```python
from build123d import *

# Parameters (mm, degrees)
BOSS_EXTRUDE1_DEPTH      = 6.35
FILLET1_R                = 12.7
CUT_EXTRUDE2_DEPTH       = 3.175
BOSS_EXTRUDE2_DEPTH      = 3.175
BOSS_EXTRUDE2_DEPTH_BACK = 36.135303
SKETCH4_R                = 9.525
SKETCH4_R_2              = 6.35
SKETCH5_R                = 9.525
SKETCH5_R_2              = 6.35
BOSS_EXTRUDE3_DEPTH      = 25.4
CHAMFER2_SIZE            = 1
CHAMFER4_SIZE            = 1


with BuildPart() as part:
    # Sketch1 → Boss-Extrude1 (new, symmetric)
    with BuildSketch(Plane.YZ):
        Polygon((-25.4, 10.735303163), (0, 25.4), (25.4, 25.4), (25.4, -25.4), (-25.4, -25.4), align=None)
    extrude(amount=BOSS_EXTRUDE1_DEPTH, both=True)

    # Fillet1
    fillet1_edges = [part.edges().sort_by_distance(p)[0] for p in [
        (0, 25.4, -25.4),
    ]]
    fillet(fillet1_edges, radius=FILLET1_R)

    # Sketch3 → Cut-Extrude2 (cut)
    with BuildSketch(Plane.YZ.offset(6.35)):
        with BuildLine():
            Line((-22.225, -22.225), (12.7, -22.225))
            ThreePointArc((12.7, -22.225), (19.435192091, -19.435192091), (22.225, -12.7))
            Line((22.225, -12.7), (22.225, 22.225))
            Line((22.225, 22.225), (0.850738686, 22.225))
            Line((0.850738686, 22.225), (-22.225, 8.902216058))
            Line((-22.225, 8.902216058), (-22.225, -22.225))
        make_face()
    cut_extrude2 = extrude(amount=-CUT_EXTRUDE2_DEPTH, mode=Mode.SUBTRACT)

    # Mirror1: Cut-Extrude2 across plane
    add(cut_extrude2.mirror(Plane(origin=(0, 0, 0), x_dir=(0, 0, 1), z_dir=(1, 0, 0))), mode=Mode.SUBTRACT)

    # Sketch4 → Boss-Extrude2 (add, two sides: drawn at the far end of the back side and taken through both)
    with BuildSketch(Plane(origin=(0, 0, -25.4), x_dir=(1, 0, 0), z_dir=(0, 0, -1)).offset(-BOSS_EXTRUDE2_DEPTH_BACK)):
        with Locations(Location((0, 33.02, 0), (0, 0, 233.130102354))):
            Circle(SKETCH4_R)
        with Locations(Location((0, 33.02, 0), (0, 0, 270))):
            Circle(SKETCH4_R_2, mode=Mode.SUBTRACT)
    extrude(amount=BOSS_EXTRUDE2_DEPTH + BOSS_EXTRUDE2_DEPTH_BACK)

    # Sketch5 → Boss-Extrude3 (add)
    with BuildSketch(Plane(origin=(0, 25.4, 0), x_dir=(-1, 0, 0), z_dir=(0, 1, 0))):
        with Locations((0, 33.02)):
            Circle(SKETCH5_R)
        with Locations(Location((0, 33.02, 0), (0, 0, 90))):
            Circle(SKETCH5_R_2, mode=Mode.SUBTRACT)
    extrude(amount=-BOSS_EXTRUDE3_DEPTH)

    # Chamfer2
    # the kernel refuses this chamfer: 1 mm, written as the material it takes off along each edge
    with BuildSketch(Plane(origin=(0, -33.02, 10.735303), x_dir=(0.3638595085405839, 0.931453841070294, 0), z_dir=(-0.931453841070294, 0.3638595085405839, 0))) as chamfer2_piece_1_section:
        Polygon((9.525, CHAMFER2_SIZE), (9.525 - CHAMFER2_SIZE, 0), (9.525, 0), align=None)
    chamfer2_piece_1 = revolve(axis=Axis((0, -33.02, 10.735303), (0, 0, -1)), revolution_arc=317.325176487, mode=Mode.PRIVATE)
    chamfer2_piece_1 = split(chamfer2_piece_1, bisect_by=Plane(origin=(5.777045626, -25.4, 10.24862198), z_dir=(0, -1, 0)), keep=Keep.TOP, mode=Mode.PRIVATE)
    add(chamfer2_piece_1, mode=Mode.SUBTRACT)
    with BuildSketch(Plane(origin=(0, -33.02, -28.575), x_dir=(-0.6000000000021781, 0.7999999999983665, 0), z_dir=(-0.7999999999983665, -0.6000000000021781, 0))) as chamfer2_piece_2:
        Polygon((9.525, -CHAMFER2_SIZE), (9.525 - CHAMFER2_SIZE, 0), (9.525, 0), align=None)
    revolve(axis=Axis((0, -33.02, -28.575), (0, 0, -1)), mode=Mode.SUBTRACT)
    with BuildSketch(Plane(origin=(0, 25.4, 33.02), x_dir=(-0.3638595085405501, 0, -0.9314538410703074), z_dir=(0.9314538410703074, 0, -0.3638595085405501))) as chamfer2_piece_3_section:
        Polygon((9.525, -CHAMFER2_SIZE), (9.525 - CHAMFER2_SIZE, 0), (9.525, 0), align=None)
    chamfer2_piece_3 = revolve(axis=Axis((0, 25.4, 33.02), (0, 1, 0)), revolution_arc=317.325176487, mode=Mode.PRIVATE)
    chamfer2_piece_3 = split(chamfer2_piece_3, bisect_by=Plane(origin=(0, 24.920234358, 25.4), z_dir=(0, 0, 1)), keep=Keep.TOP, mode=Mode.PRIVATE)
    add(chamfer2_piece_3, mode=Mode.SUBTRACT)
    with BuildSketch(Plane(origin=(0, 0, 33.02), x_dir=(-0.3638595085405531, 0, -0.9314538410703063), z_dir=(0.9314538410703063, 0, -0.3638595085405531))) as chamfer2_piece_4_section:
        Polygon((9.525, CHAMFER2_SIZE), (9.525 - CHAMFER2_SIZE, 0), (9.525, 0), align=None)
    chamfer2_piece_4 = revolve(axis=Axis((0, 0, 33.02), (0, 1, 0)), revolution_arc=317.325176487, mode=Mode.PRIVATE)
    chamfer2_piece_4 = split(chamfer2_piece_4, bisect_by=Plane(origin=(-5.452412952, 0.490850729, 25.4), z_dir=(0, 0, 1)), keep=Keep.TOP, mode=Mode.PRIVATE)
    add(chamfer2_piece_4, mode=Mode.SUBTRACT)

    # Sweep3: sweep along a path in Sketch6
    with BuildLine(Plane.YZ) as sweep3_path:
        Line((0, 33.02), (-20.32, 33.02))
        ThreePointArc((-20.32, 33.02), (-29.300256121, 29.300256121), (-33.02, 20.32))
        Line((-33.02, 20.32), (-33.02, 10.735303163))
    # Sketch7 → Sweep3 (sweep)
    with BuildSketch(Plane.XZ):
        with BuildLine():
            Line((-8.525, 33.02), (-6.35, 33.02))
            ThreePointArc((-6.35, 33.02), (0, 26.67), (6.35, 33.02))
            Line((6.35, 33.02), (8.525, 33.02))
            ThreePointArc((8.525, 33.02), (0, 24.495), (-8.525, 33.02))
        make_face()
    sweep(path=sweep3_path.line)

    # Chamfer4
    chamfer4_edges = [part.edges().sort_by_distance(p)[0] for p in [
        (3.175, -22.225, -6.661391971),
        (3.175, -10.687130657, 15.563608029),
        (3.175, 11.537869343, 22.225),
        (3.175, 22.225, 4.7625),
        (3.175, 19.435192091, -19.435192091),
        (3.175, -4.7625, -22.225),
        (-3.175, -22.225, -6.661391971),
        (-3.175, -4.7625, -22.225),
        (-3.175, 19.435192091, -19.435192091),
        (-3.175, 22.225, 4.7625),
        (-3.175, 11.537869343, 22.225),
        (-3.175, -10.687130657, 15.563608029),
    ]]
    chamfer(chamfer4_edges, length=CHAMFER4_SIZE)


solid = part.part
```
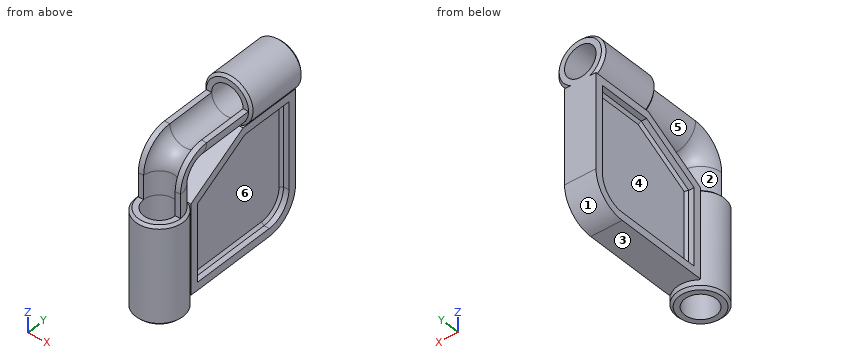
The listing builds one solid part. Answer for the finished solid, in the listing's coordinates (mm). Face numbers are marked on the shaded views. A direction names the side the tool comes from. Coordinates: 2 decimals unless noted, no trailing zeros. Write each loop counter-clockwise with the first axis right and the second up, starting at its lowest first coordinate (ties: lowest second). Pieces come first, ordered by that corner, then holes. Notation, with made-up numbers: (-17, 3) - (21, 3) arc R32 cw to (21, 38) - close; hole circle Ø9 at (56.5, -33.75). An arc over 180 degrees is marked (long way). Return JSON: item names as keys, results as strings. Group by question number.
Q1. The part is cut by section A-A on x = 0. State how many separate pieces and enclosed holes the cut face has, and give its area (3 significant figures).
Q2. For a pull along Y with two mould halves and no side action, classify the marked faces 1, 2 and 3 as +Y half, -Y half, draft (parallel to the pull), parting line (faces both ways), or undercut.
Q3. Find the intervals of material crossed by line 1 along Z through (x, y) = (0, 9) (3 decimals); line 2 along Y through (x, z) = (5, -8.5) (3 decimals); line 3 along X through (y, z) = (-33.02, -13.5) (3 decimals), in increasing order. Write a range as [from, to].
Q4. The part is cut by section B-B on z = 6. Write down the section's boundary in (x, y) (3 decimals).
Q5. Which of the six approach directions +Z, -Z, +X, -X, +Y, -Y give full straight-line access (tool end or side, diameter ignored) to the marked faces 4, 5 and 6?
Q6. The part is cut by section D-D on y = 3. Write down the section's boundary in (x, z) (3 decimals).
Q7. Flat-ended cylindrical pins translate along their axes: pin 1 Ø6 at (y, z) = (12.5, 22.5) entering from +X; pin 2 Ø2 at (x, z) = (-5, -15) entering from -Y; pin 3 Ø8 at (y, z) = (-14, 4) entering from -X (3 decimals); pin 4 Ø1.5 at (y, z) = (-16.5, 19) entering from +X. Find the tip coordinate at first contact, or state that the pin passes through.
Q8. The part is cut by section C-C on y = -13. Write down the section's boundary in (x, z) (3 decimals), and give its area (3 significant figures).
Evaluation:
{
 "1": {"separate pieces": "3", "enclosed holes": "1", "area": "2,730 mm2"},
 "2": {"face 1": "+Y half", "face 2": "undercut", "face 3": "draft"},
 "3": {"line 1": "z = [-25.4, 26.67], [39.37, 42.545]", "line 2": "y = [-41.127, -36.934], [-29.106, -22.225], [22.225, 25.4]", "line 3": "x = [-9.525, -6.35], [6.35, 9.525]"},
 "4": {"outline": "(-6.35, -25.4) - (-5.715, -25.4) arc R9.525 ccw (long way) to (5.715, -25.4) - (6.35, -25.4) - (6.35, -22.225) - (4.175, -22.225) - (3.175, -21.225) - (3.175, 21.225) - (4.175, 22.225) - (6.35, 22.225) - (6.35, 25.4) - (-6.35, 25.4) - (-6.35, 22.225) - (-4.175, 22.225) - (-3.175, 21.225) - (-3.175, -21.225) - (-4.175, -22.225) - (-6.35, -22.225) - close; hole circle Ø12.7 at (0, -33.02)"},
 "5": {"face 4": "-X", "face 5": "none", "face 6": "+X"},
 "6": {"outline": "(-6.35, -25.4) - (6.35, -25.4) - (6.35, -22.225) - (4.175, -22.225) - (3.175, -21.225) - (3.175, 21.225) - (4.175, 22.225) - (6.35, 22.225) - (6.35, 25.4) - (5.715, 25.4) arc R9.525 ccw (long way) to (-5.715, 25.4) - (-6.35, 25.4) - (-6.35, 22.225) - (-4.175, 22.225) - (-3.175, 21.225) - (-3.175, -21.225) - (-4.175, -22.225) - (-6.35, -22.225) - close; hole circle Ø12.7 at (0, 33.02)"},
 "7": {"pin 1": "stops at x = 6.35", "pin 2": "stops at y = -41.66", "pin 3": "stops at x = -3.175", "pin 4": "passes through"},
 "8": {"outline": "(-8.525, 33.02) arc R8.525 ccw to (8.525, 33.02) - (6.35, 33.02) arc R6.35 cw to (-6.35, 33.02) - close; (-6.35, -25.4) - (6.35, -25.4) - (6.35, -22.225) - (4.175, -22.225) - (3.175, -21.225) - (3.175, 13.074) - (4.175, 14.228) - (6.35, 14.228) - (6.35, 17.894) - (-6.35, 17.894) - (-6.35, 14.228) - (-4.175, 14.228) - (-3.175, 13.074) - (-3.175, -21.225) - (-4.175, -22.225) - (-6.35, -22.225) - close", "area": "371 mm2"}
}
